Autodesk Inventor part; units mm, degrees
ref_plane "工作平面1" through (0, 0, 0) normal (0, 0, 1) x (1, 0, 0)
ref_plane "工作平面2" through (50, 0, 3) normal (0, 0, -1) x (-1, 0, 0)
ref_plane "YZ Plane" through (0, 0, 0) normal (1, 0, 0) x (0, 1, 0)
ref_plane "工作平面1" through (0, 0, 0) normal (0, 0, 1) x (1, 0, 0)
sketch "草图1" plane through (0, 0, 0) normal (0, 0, 1) x (1, 0, 0)
  arc A0 (50, 75) -> (50, -75) centre (50, 0) ccw construction
  line L0 (50, 75) -> (50, 100) construction
  arc A1 (50, 100) -> (50, -100) centre (50, 0) ccw construction
  line L1 (50, -100) -> (50, -75) construction
  circle A2 centre (50, 0) radius 100
  circle A3 centre (50, 0) radius 87.5 construction
  line L2 (190.8101, 0) -> (-90.8101, 0) construction
  circle A4 centre (137.5, 0) radius 5.5
  circle A5 centre (93.75, 75.7772) radius 5.5
  circle A6 centre (6.25, 75.7772) radius 5.5
  circle A7 centre (-37.5, 0) radius 5.5
  circle A8 centre (6.25, -75.7772) radius 5.5
  circle A9 centre (93.75, -75.7772) radius 5.5
  point P0 (0, 0)
  dimension "d0" = 175
  dimension "d1" = 11
  dimension "d4" = 360
extrude "拉伸1" add sketch "草图1" along normal blind 12
sketch "草图2" plane through (50, 0, 12) normal (0, 0, 1) x (1, 0, 0)
  circle A0 centre (0, 0) radius 48 construction
  circle A1 centre (0, 0) radius 48.5
  point P0 (-50, 0)
  dimension "d19" = 97
extrude "拉伸2" cut sketch "草图2" against normal up to surface (12 mm away)
sketch "草图3" plane through (50, 0, 0) normal (0, 0, -1) x (-1, 0, 0)
  circle A0 centre (0, 0) radius 100
  circle A1 centre (0, 0) radius 75
  circle A2 centre (0, 0) radius 70
  point P0 (50, 0)
  dimension "d11" = 150
  dimension "d12" = 140
extrude "拉伸3" add sketch "草图3" along normal blind 38 contours A1
sketch "草图4" plane through (50, 0, 12) normal (0, 0, 1) x (1, 0, 0)
  circle A0 centre (0, 0) radius 48.5 construction
  circle A1 centre (0, 0) radius 75
  point P0 (-50, 0)
  dimension "d15" = 150
extrude "拉伸4" cut sketch "草图4" against normal blind 1
fillet "圆角1" radius 1 1 edges at (-25, 0, 11)
sketch "草图5" plane through (50, 0, 0) normal (0, 0, -1) x (-1, 0, 0)
  circle A0 centre (0, 0) radius 70
  circle A1 centre (0, 0) radius 48.5
  point P0 (50, 0)
extrude "拉伸5" add sketch "草图5" along normal blind 5
ref_plane "工作平面2" through (50, 0, 3) normal (0, 0, -1) x (-1, 0, 0)
sketch "草图6" plane through (50, 0, 3) normal (0, 0, -1) x (-1, 0, 0)
  circle A0 centre (0, 0) radius 48.5 construction
  circle A1 centre (0, 0) radius 49.275
  point P0 (50, 0)
  dimension "d22" = 98.55
extrude "拉伸6" cut sketch "草图6" against normal mid plane 3.55
sketch "草图7" plane through (50, 0, 0) normal (0, 0, -1) x (-1, 0, 0)
  circle A0 centre (0, 0) radius 48.5 construction
  circle A1 centre (0, 0) radius 75
  circle A2 centre (0, 0) radius 74
  point P0 (50, 0)
  dimension "d25" = 1
extrude "拉伸7" cut sketch "草图7" along normal blind 2
properties part number "轴承通盖"
The model under review builds one solid part; all positions refer to its coordinate system, in mm. A direction names the side the tool comes from. Give positions to 0.01 mm unless a question says otherwise; leave off trailing zeros. Loops run counter-clockwise (first coordinate to the right, second up) from the corner with the lowest first, then second, coordinate; pieces in that order, holes last. Notation, with made-up numbers: (-25, -15) -> (29, -15) arc R13 cw to (29, 1) -> close; hole circle Ø9 at (2.5, -33). An arc over 180 degrees is marked (long way). Answer as a JSON object with one key per item and string values. Group by question number.
Q1. Take a section at D-D (x = -37.5). Write out the cut boundary in (y, z), plus the area to 3 significant figures.
Q2. Wall thickness on line 1 along Y through (x, z) = (93.75, 7.75); line 2 along X through (y, z) = (-79.5, 7); line 3 along Y through (x, z) = (6.25, 2.5): over which ranges is each line inside the solid? List them lowest first.
Q3. Take a section at B-B (z = -33.5). Write out the cut boundary in (x, y), plus the area to 3 significant figures.
Q4. Insertion check: pin 1 (12.5 mm diameter, centred on x = 6.25, y = 75.78, fed in from -Z); pin 2 (9 mm diameter, centred on x = 93.75, y = -75.78, fed in from +Z); pin 3 (2 mm diameter, centred on x = 31, z = -2, fed in from -Y); pin 4 (12 mm diameter, centred on x = 90, y = -39.5, fed in from +Z). Each pin has a flat end and moves straight along its axis. Give the tip position at first contact, or say it passes through.
Q5. Tool access review of faces 1 (the flat face through (98, -15, 11)), 2 (the flat face through (67, -46, -5)), 3 (the flat face through (-5, -50, -2)): name each direction out of +Z, -Z, +X, -X, +Y, -Y from which nothing blocks a thin tool from reaching the whole face with its end or side.
Q6. Draft analysis for pull direction Y (two halves, no side actions). For faces 4 (the flat face through (50, 75, 0)), 5 (the cylindrical face through (132, 0, 6)), 6 (the cylindrical face through (145.38, -30.04, 5.92)), state which applies: pulls with the +Y half, pulls with the -Y half, needs draft (parallel to the pull), parting line crosses it, or undercut.
Q7. Take a section at C-C (y = 0). State how many separate pieces and enclosed holes the cut face has, plus the area to 3 significant figures.
Answer below:
{
 "1": {"outline": "(-48.41, 0) -> (-5.5, 0) -> (-5.5, 12) -> (-48.41, 12) -> close; (5.5, 0) -> (48.41, 0) -> (48.41, 12) -> (5.5, 12) -> close", "area": "1,030 mm2"},
 "2": {"line 1": "y = -89.92 to -81.28, -70.28 to -20.93, 20.93 to 70.28, 81.28 to 89.92", "line 2": "x = -10.66 to 2.2, 10.3 to 89.7, 97.8 to 110.66", "line 3": "y = -89.92 to -81.28, -70.28 to -22.67, 22.67 to 70.28, 81.28 to 89.92"},
 "3": {"outline": "circle Ø150 at (50, 0); hole circle Ø140 at (50, 0)", "area": "2,280 mm2"},
 "4": {"pin 1": "stops at z = 0", "pin 2": "passes through", "pin 3": "stops at y = -72.81", "pin 4": "stops at z = 11"},
 "5": {"face 1": "+Z", "face 2": "-Z", "face 3": "none"},
 "6": {"face 4": "needs draft", "face 5": "undercut", "face 6": "parting line crosses it"},
 "7": {"separate pieces": "4", "enclosed holes": "0", "area": "1,500 mm2"}
}
